```python
from build123d import *

# Parameters (mm, degrees)
F0_W     = 203.2
F0_H     = 165.1
F1_DEPTH = 4.3434
F3_DEPTH = 4.3434
F4_W     = 4.3434
F4_H     = 12.7
F5_DEPTH = 4.3434


with BuildPart() as f1:
    # F0 (on Top) → F1 (new body)
    with BuildSketch(Plane.XY):
        with Locations((45.995247, 32.638061)):
            Rectangle(F0_W, F0_H)
    extrude(amount=-F1_DEPTH)

    # F2 (on Top) → F3 (join)
    with BuildSketch(Plane.XY):
        Polygon((-4.896646, -49.593655), (-11.246646, -49.593655), (-11.246646, -53.937055), (-4.896646, -53.937055), (1.453354, -53.937055), (1.453354, -49.593655), align=None)
        Polygon((103.053354, -53.937055), (103.053354, -49.593655), (96.703354, -49.593655), (90.353354, -49.593655), (90.353354, -53.937055), (96.703354, -53.937055), align=None)
    extrude(amount=-F3_DEPTH)

    # F4 (on Top) → F5 (join)
    with BuildSketch(Plane.XY):
        with Locations((-57.213607, 32.638061)):
            Rectangle(F4_W, F4_H)
        with Locations((149.000803, 32.638061)):
            Rectangle(F4_W, F4_H)
    extrude(amount=-F5_DEPTH)


solid = f1.part
```
Here's how the part is built. I have some questions about the finished solid (model axes, mm). A direction names the side the tool comes from. Round coordinates to 2 decimals unless told otherwise and drop trailing zeros. Write each loop counter-clockwise with the first axis right and the second up, starting at its lowest first coordinate (ties: lowest second). Pieces come first, ordered by that corner, then holes.
Q1. If we section it at C-C on x = 79: Write out the boundary of the cut face in (y, z).
Q2. Which directions (+Z, -Z, +X, -X, +Y, -Y) give clear straight access to the entire face, cutting with the end or side of a thin tool? Please do faces 1 (the flat face through (-55.605, 77, -2)), 2 (the flat face through (147.595, -12, -2)), 3 (the flat face through (-34, -49.912, -2)), 4 (the flat face through (97, -53.937, -2)).
Q3. If we mould it in two halves opening along X, with no side actions, what happens to faces 5 (the flat face through (147.595, 77, -2)), 6 (the flat face through (45, -49.912, -2)), 7 (the flat face through (44, 32, -4.343))? For each: +X half, -X half, draft (parallel to the pull), parting line (faces both ways), or undercut.
Q4. If we section it at B-B on y = 92: Write out the boundary of the cut face in (x, z).
Q5. Will these pins go through, and if not, where does the flat tip stop? P1, Ø2, axis at y = -26.5, z = -2.5, coming from the -X side; P2, Ø2, axis at x = 56, z = -1.5, coming from the -Y side; P3, Ø1.9, axis at x = -58, z = -2.5, coming from the -Y side.
Q6. Please list where these lines run through material, in increasing order: probe 1 along Y at (x, z) = (138, -4.1); probe 2 along X at (y, z) = (84, -1.95).
Q7. If we section it at A-A on z = -1.05: Write out the boundary of the cut face in (x, y), plus the area to 3 significant figures.
Answer below:
1. outline: (-49.91, -4.34) - (115.19, -4.34) - (115.19, 0) - (-49.91, 0) - close
2. face 1: +Z, -Z, -X, +Y
2. face 2: +Z, -Z, +X, -Y
2. face 3: +Z, -Z, -X, -Y
2. face 4: +Z, -Z, +X, -X, -Y
3. face 5: +X half
3. face 6: undercut
3. face 7: draft
4. outline: (-55.6, -4.34) - (147.6, -4.34) - (147.6, 0) - (-55.6, 0) - close
5. P1: stops at x = -55.6
5. P2: stops at y = -49.91
5. P3: stops at y = 26.29
6. probe 1: y = -49.91 to 115.19
6. probe 2: x = -55.6 to 147.6
7. outline: (-59.39, 26.29) - (-55.6, 26.29) - (-55.6, -49.91) - (-11.25, -49.91) - (-11.25, -53.94) - (1.45, -53.94) - (1.45, -49.91) - (90.35, -49.91) - (90.35, -53.94) - (103.05, -53.94) - (103.05, -49.91) - (147.6, -49.91) - (147.6, 26.29) - (151.17, 26.29) - (151.17, 38.99) - (147.6, 38.99) - (147.6, 115.19) - (-55.6, 115.19) - (-55.6, 38.99) - (-59.39, 38.99) - close
7. area: 33,700 mm2
